Input: part model. Units: mm. Frame: model coordinates. Face numbers are marked on the shaded views. A direction names the side the tool comes from. Round coordinates to 2 decimals unless told otherwise and drop trailing zeros. Order: outer loops, then holes, each group sorted by start corner. A loop starts at its lowest first (then second) coordinate and runs counter-clockwise, first axis right, second up. Notation, with made-up numbers: (16, 62.25) -> (71, 62.25) arc R15 ccw to (71, 83.25) -> close; hole circle Ø6 at (70, 72). An arc over 180 degrees is marked (long way). Use a Markdown table: item, result.
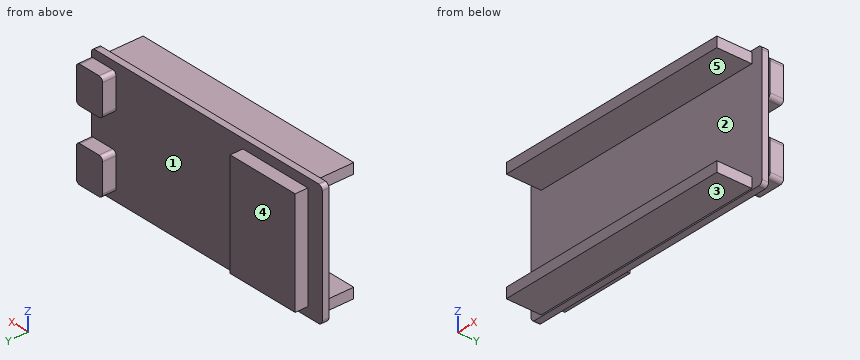
from build123d import *

# Parameters (mm, degrees)
BOARD_START   = 12.5
BOARD_DEPTH   = 1.6
WROOM_START   = 14.1
SKETCH2_W     = 18
SKETCH2_H     = 25.5
WROOM_DEPTH   = 3.1
USB_C_START   = 14.1
USB_C_DEPTH   = 3.3
HEADERS_START = 4
SKETCH4_W     = 58.4
SKETCH4_H     = 2.5
HEADERS_DEPTH = 8.5


with BuildPart() as part:
    # Sketch1 → Board (new body)
    with BuildSketch(Plane(origin=(0, 0, 0), x_dir=(1, 0, 0), z_dir=(0, 1, 0)).offset(BOARD_START)):
        with BuildLine():
            Line((-18, -20), (44, -20))
            ThreePointArc((44, -20), (44.707106781, -20.292893219), (45, -21))
            Line((45, -21), (45, -49))
            ThreePointArc((45, -49), (44.707106781, -49.707106781), (44, -50))
            Line((44, -50), (-18, -50))
            ThreePointArc((-18, -50), (-18.707106781, -49.707106781), (-19, -49))
            Line((-19, -49), (-19, -21))
            ThreePointArc((-19, -21), (-18.707106781, -20.292893219), (-18, -20))
        make_face()
    extrude(amount=BOARD_DEPTH)

    # Sketch2 → WROOM (add)
    with BuildSketch(Plane(origin=(0, 0, 0), x_dir=(1, 0, 0), z_dir=(0, 1, 0)).offset(WROOM_START)):
        with Locations((-6, -35)):
            Rectangle(SKETCH2_W, SKETCH2_H)
    extrude(amount=WROOM_DEPTH)

    # Sketch3 → USB-C (add)
    with BuildSketch(Plane(origin=(0, 0, 0), x_dir=(1, 0, 0), z_dir=(0, 1, 0)).offset(USB_C_START)):
        with BuildLine():
            Line((39.15, -22), (44.45, -22))
            ThreePointArc((44.45, -22), (45.157106781, -22.292893219), (45.45, -23))
            Line((45.45, -23), (45.45, -29.94))
            ThreePointArc((45.45, -29.94), (45.157106781, -30.647106781), (44.45, -30.94))
            Line((44.45, -30.94), (39.15, -30.94))
            ThreePointArc((39.15, -30.94), (38.442893219, -30.647106781), (38.15, -29.94))
            Line((38.15, -29.94), (38.15, -23))
            ThreePointArc((38.15, -23), (38.442893219, -22.292893219), (39.15, -22))
        make_face()
        with BuildLine():
            Line((39.15, -39.06), (44.45, -39.06))
            ThreePointArc((44.45, -39.06), (45.157106781, -39.352893219), (45.45, -40.06))
            Line((45.45, -40.06), (45.45, -47))
            ThreePointArc((45.45, -47), (45.157106781, -47.707106781), (44.45, -48))
            Line((44.45, -48), (39.15, -48))
            ThreePointArc((39.15, -48), (38.442893219, -47.707106781), (38.15, -47))
            Line((38.15, -47), (38.15, -40.06))
            ThreePointArc((38.15, -40.06), (38.442893219, -39.352893219), (39.15, -39.06))
        make_face()
    extrude(amount=USB_C_DEPTH)

    # Sketch4 → Headers (add)
    with BuildSketch(Plane(origin=(0, 0, 0), x_dir=(1, 0, 0), z_dir=(0, 1, 0)).offset(HEADERS_START)):
        with Locations((13, -21.6)):
            Rectangle(SKETCH4_W, SKETCH4_H)
        with Locations((13, -48.4)):
            Rectangle(SKETCH4_W, SKETCH4_H)
    extrude(amount=HEADERS_DEPTH)


solid = part.part
1) Line query: L1, parallel to Z at x = -10.5, y = 4.75; L2, parallel to X at y = 15, z = 24. Output: solid intervals per line, ascending. Write a range as [from, to].
Results found:
| item | result |
|---|---|
| L1 | z = [20.35, 22.85], [47.15, 49.65] |
| L2 | x = [-15, 3], [38.15, 45.45] |
2) Cut plane D-D on x = -8. Return loops of the section in (y, z).
Results found:
| item | result |
|---|---|
| outline | (4, 20.35) -> (12.5, 20.35) -> (12.5, 20) -> (14.1, 20) -> (14.1, 22.25) -> (17.2, 22.25) -> (17.2, 47.75) -> (14.1, 47.75) -> (14.1, 50) -> (12.5, 50) -> (12.5, 49.65) -> (4, 49.65) -> (4, 47.15) -> (12.5, 47.15) -> (12.5, 22.85) -> (4, 22.85) -> close |
3) Cut plane B-B on x = 41. Return loops of the section in (y, z).
Results found:
| item | result |
|---|---|
| outline | (4, 20.35) -> (12.5, 20.35) -> (12.5, 20) -> (14.1, 20) -> (14.1, 22) -> (17.4, 22) -> (17.4, 30.94) -> (14.1, 30.94) -> (14.1, 39.06) -> (17.4, 39.06) -> (17.4, 48) -> (14.1, 48) -> (14.1, 50) -> (12.5, 50) -> (12.5, 49.65) -> (4, 49.65) -> (4, 47.15) -> (12.5, 47.15) -> (12.5, 22.85) -> (4, 22.85) -> close |
4) Pin query (flat end, axial travel): pin 1 Ø6 at (x, y) = (-11.5, 7.5) entering from +Z; pin 2 Ø1 at (y, z) = (16, 43.5) entering from -X; pin 3 Ø4 at (x, z) = (-0.5, 45) entering from -Y. Return the tip coordinate at first contact, or that it passes through.
Results found:
| item | result |
|---|---|
| pin 1 | stops at z = 49.65 |
| pin 2 | stops at x = -15 |
| pin 3 | stops at y = 12.5 |
5) Pull-direction query (X, two-part tool) for the marked faces 1 and 2; classes: +X half, -X half, draft (parallel to the pull), parting line (faces both ways), or undercut.
Results found:
| item | result |
|---|---|
| face 1 | undercut |
| face 2 | draft |
6) Set-up query: the marked faces 3, 4 and 5. Return all of +Z, -Z, +X, -X, +Y, -Y with unobstructed straight access to the full face (end or side cutting, diameter ignored); none if empty.
Results found:
| item | result |
|---|---|
| face 3 | -Z, +X, -X, -Y |
| face 4 | +Z, -Z, -X, +Y |
| face 5 | +X, -X, -Y |
7) Cut plane C-C on z = 37. Return loops of the section in (x, y), and give its area (3 significant figures).
Results found:
| item | result |
|---|---|
| outline | (-19, 12.5) -> (45, 12.5) -> (45, 14.1) -> (3, 14.1) -> (3, 17.2) -> (-15, 17.2) -> (-15, 14.1) -> (-19, 14.1) -> close |
| area | 158 mm² |
8) Cut plane A-A on y = 5.5. Return loops of the section in (x, z), and give its area (3 significant figures).
Results found:
| item | result |
|---|---|
| outline | (-16.2, 20.35) -> (42.2, 20.35) -> (42.2, 22.85) -> (-16.2, 22.85) -> close; (-16.2, 47.15) -> (42.2, 47.15) -> (42.2, 49.65) -> (-16.2, 49.65) -> close |
| area | 292 mm² |
